from build123d import *
from build123d import SkipClean  # not in build123d's __all__

# Parameters (mm, degrees)
F0_W      = 15
F0_H      = 15
F0_H_2    = 6
F1_DEPTH  = 10
F2_R      = 1.5
F3_DEPTH  = 2
F5_DEPTH  = 1
F6_R      = 1.5
F7_DEPTH  = 2
F8_W      = 15
F8_H      = 21
F9_DEPTH  = 7
F10_W     = 15
F10_H     = 3
F11_DEPTH = 5
F12_W     = 15
F12_H     = 5
F13_DEPTH = 3
F15_DEPTH = 25
F16_R     = 0.5


# Not quite as in the source:
# - after a boolean that leaves OpenCascade's solid faulty, fix() repairs it


with BuildPart() as f1:
    # F0 (on Front) → F1 (new body)
    with BuildSketch(Plane.XZ):
        Rectangle(F0_W, F0_H)
        with Locations((0, 10.5)):
            Rectangle(F0_W, F0_H_2)
    extrude(amount=F1_DEPTH)

    # F2 (on face) → F3 (join)
    with BuildSketch(Plane.XZ.offset(10)):
        with Locations((-3, 3)):
            Circle(F2_R)
        with Locations((-3, -3)):
            Circle(F2_R)
        with Locations((3, -3)):
            Circle(F2_R)
        with Locations((3, 3)):
            Circle(F2_R)
    extrude(amount=F3_DEPTH)

    # F4 (on face) → F5 (cut)
    with BuildSketch(Plane.XZ.offset(10)):
        with BuildLine():
            Line((-7.5, 13.5), (-7.5, 7.5))
            Line((-7.5, 7.5), (-4.2426406871, 7.5))
            ThreePointArc((-4.2426406871, 7.5), (-3.6742346142, 11.5980762114), (0, 13.5))
            Line((0, 13.5), (-7.5, 13.5))
        make_face()
        with BuildLine():
            ThreePointArc((0, 13.5), (-3.6742346142, 11.5980762114), (-4.2426406871, 7.5))
            Line((-4.2426406871, 7.5), (0, 7.5))
            Line((0, 7.5), (4.2426406871, 7.5))
            ThreePointArc((4.2426406871, 7.5), (4.4351935184, 8.2390410957), (4.5, 9))
            ThreePointArc((4.5, 9), (3.1819805153, 12.1819805153), (0, 13.5))
        make_face()
        with BuildLine():
            ThreePointArc((1.5, 9), (1.0606601718, 7.9393398282), (0, 7.5))
            ThreePointArc((0, 7.5), (-1.0606601718, 10.0606601718), (1.5, 9))
        make_face(mode=Mode.SUBTRACT)
        with BuildLine():
            Line((0, 7.5), (-4.2426406871, 7.5))
            ThreePointArc((-4.2426406871, 7.5), (0, 4.5), (4.2426406871, 7.5))
            Line((4.2426406871, 7.5), (0, 7.5))
        make_face()
        with BuildLine():
            Line((7.5, 13.5), (0, 13.5))
            ThreePointArc((0, 13.5), (3.1819805153, 12.1819805153), (4.5, 9))
            ThreePointArc((4.5, 9), (4.4351935184, 8.2390410957), (4.2426406871, 7.5))
            Line((4.2426406871, 7.5), (7.5, 7.5))
            Line((7.5, 7.5), (7.5, 13.5))
        make_face()
    extrude(amount=-F5_DEPTH, mode=Mode.SUBTRACT)

    # F6 (on face) → F7 (join)
    with BuildSketch(Plane.XZ.offset(10)):
        with Locations((0, 9)):
            Circle(F6_R)
    with SkipClean():  # cleaning this boolean's faces spoils the solid; the shape is the same uncleaned
        extrude(amount=F7_DEPTH)

    # F8 (on face) → F9 (cut)
    with BuildSketch(Plane(origin=(0, 0, 0), x_dir=(-1, 0, 0), z_dir=(0, 1, 0))):
        with Locations((0, 3)):
            Rectangle(F8_W, F8_H)
    extrude(amount=-F9_DEPTH, mode=Mode.SUBTRACT)

    add(f1.part.fix(), mode=Mode.REPLACE)

    # F10 (on face) → F11 (join)
    with BuildSketch(Plane(origin=(0, 0, -7.5), x_dir=(1, 0, 0), z_dir=(0, 0, -1))):
        with Locations((0, 8.5)):
            Rectangle(F10_W, F10_H)
    extrude(amount=F11_DEPTH)

    # F12 (on face) → F13 (join)
    with BuildSketch(Plane(origin=(0, -7, 0), x_dir=(-1, 0, 0), z_dir=(0, 1, 0))):
        with Locations((0, -10)):
            Rectangle(F12_W, F12_H)
    extrude(amount=F13_DEPTH)

    # F14 (on face) → F15 (cut)
    with BuildSketch(Plane(origin=(0, -4, 0), x_dir=(-1, 0, 0), z_dir=(0, 1, 0))):
        with BuildLine():
            Line((-7.5, -12.5), (7.5, -12.5))
            ThreePointArc((7.5, -12.5), (0, -10.237957932), (-7.5, -12.5))
        make_face()
    extrude(amount=-F15_DEPTH, mode=Mode.SUBTRACT)

    # F16
    f16_edges = [f1.edges().sort_by_distance(p)[0] for p in [
        (-7.5, -7, -12.5),
        (7.5, -7, -12.5),
    ]]
    fillet(f16_edges, radius=F16_R)


solid = f1.part
Input: part model. Units: mm. Frame: model coordinates. A direction names the side the tool comes from. Give positions to 0.01 mm unless a question says otherwise; leave off trailing zeros. Order: outer loops, then holes, each group sorted by start corner. A loop starts at its lowest first (then second) coordinate and runs counter-clockwise, first axis right, second up. Notation, with made-up numbers: (-28.5, 10) -> (30.5, 10) arc R21 ccw to (30.5, 23) -> close; hole circle Ø3 at (65.5, -32). An arc over 180 degrees is marked (long way). Use one line per item in the form item = value.
1) Line query: probe 1 along Y at (x, z) = (-0.5, 1); probe 2 along Y at (x, z) = (6, -8.75); probe 3 along Z at (x, y) = (0, -7.25). Output: solid intervals per line, ascending.
Response values:
probe_1 = -10 to -7
probe_2 = -10 to -4
probe_3 = -10.24 to 13.5
2) Reachability of faces 4 (the flat face through (5.8, -9.5, 7.5)), 5 (the cylindrical face through (3.69, -10.99, 1.67)), 6 (the flat face through (-5.9, -9.5, 7.5)) from +Z, -Z, +X, -X, +Y, -Y: full face, straight path, thin tool, end or side. Return the list, or none.
Response values:
face_4 = +Z, +X, -Y
face_5 = -Y
face_6 = +Z, -X, -Y
3) Mould query, pull axis X, two halves, no side actions, for faces 1 (the cylindrical face through (-0.1, -9.5, 4.5)), 2 (the flat face through (0, -7, 3)), 3 (the flat face through (-7.5, -8, -2)). Classes: pulls with the +X half, pulls with the -X half, needs draft (parallel to the pull), parting line crosses it, or undercut.
Response values:
face_1 = undercut
face_2 = needs draft
face_3 = pulls with the -X half
4) Section B-B, the plane z = -3. Return loops of the section in (x, y).
Response values:
outline = (-7.5, -10) -> (-4.5, -10) -> (-4.5, -12) -> (-1.5, -12) -> (-1.5, -10) -> (1.5, -10) -> (1.5, -12) -> (4.5, -12) -> (4.5, -10) -> (7.5, -10) -> (7.5, -7) -> (-7.5, -7) -> close
5) First-contact query: pin 1 Ø0.5 at (x, y) = (6, -9.5) entering from +Z; pin 2 Ø2 at (x, z) = (3, 1) entering from -Y; pin 3 Ø1.5 at (x, y) = (-2, -10) entering from +Z; pin 4 Ø3 at (x, y) = (-1, -5) entering from -Z. Flat tips, straight axial feed; report the tip coordinate or a pass-through.
Response values:
pin_1 = 7.5
pin_2 = -12
pin_3 = 9.83
pin_4 = -10.47
6) Section D-D, the plane x = 0.25. Return loops of the section in (y, z).
Response values:
outline = (-12, 7.52) -> (-9, 7.52) -> (-9, 4.51) -> (-10, 4.51) -> (-10, -10.24) -> (-4, -10.24) -> (-4, -7.5) -> (-7, -7.5) -> (-7, 13.5) -> (-9, 13.5) -> (-9, 10.48) -> (-12, 10.48) -> close
7) Section A-A, the plane y = -9.25. Return loops of the section in (x, z).
Response values:
outline = (-7.5, -11.6) arc R0.5 ccw to (-6.75, -12.04) arc R13.56 cw to (6.75, -12.04) arc R0.5 ccw to (7.5, -11.6) -> (7.5, 7.5) -> (4.24, 7.5) arc R4.5 cw to (-4.24, 7.5) -> (-7.5, 7.5) -> close; circle Ø3 at (0, 9)
8) Section C-C, the plane y = -4.75. Return loops of the section in (x, z).
Response values:
outline = (-7.5, -11.6) arc R0.5 ccw to (-6.75, -12.04) arc R13.56 cw to (6.75, -12.04) arc R0.5 ccw to (7.5, -11.6) -> (7.5, -7.5) -> (-7.5, -7.5) -> close
